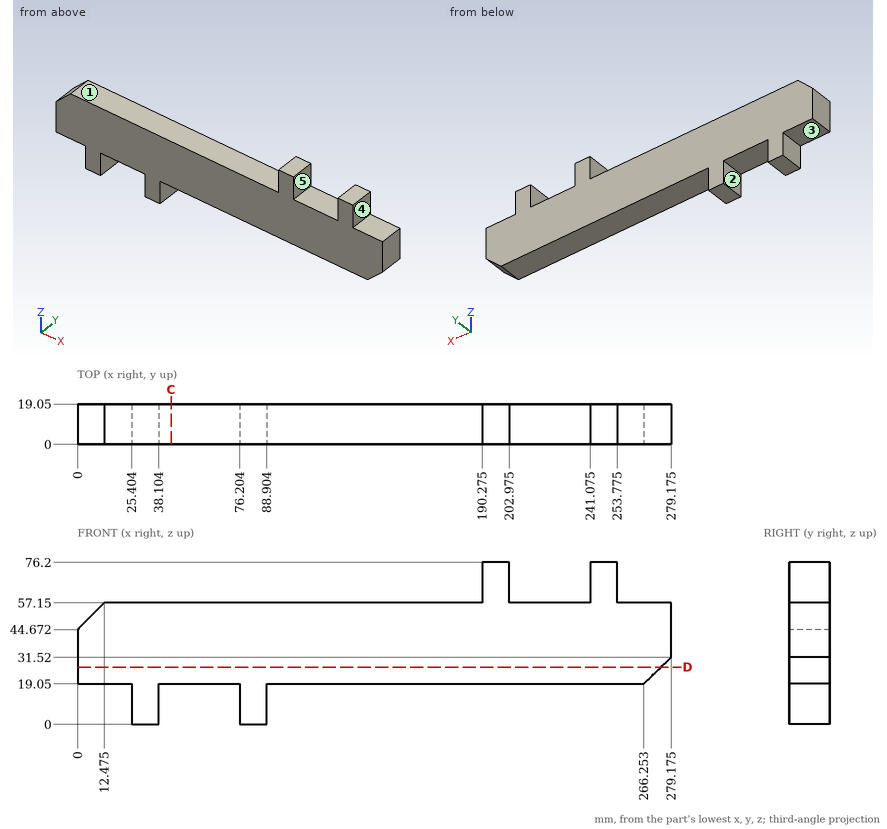
Drawing for the job (mm, zero at the part's lowest x, y, z). A direction names the side the tool comes from. Round coordinates to 2 decimals unless told otherwise and drop trailing zeros. Loops run counter-clockwise (first coordinate to the right, second up) from the corner with the lowest first, then second, coordinate; pieces in that order, holes last.
1. Band-saw the part on D-D, the plane z = 27. List the corners of the cut face in (x, y).
Check values:
outline: (0, 0) - (274.49, 0) - (274.49, 19.05) - (0, 19.05) - close
2. Drop flat-ended pins along their axis: P1, Ø9.5, axis at y = 13.5, z = 65.5, coming from the -X side (1 decimal); P2, Ø5.5, axis at x = 53.5, y = 6.5, coming from the -Z side; P3, Ø9.5, axis at y = 8.5, z = 67, coming from the +X side (1 decimal); P4, Ø5, axis at x = 101, z = 16.5, coming from the +Y side. Give the stop position or say it passes through.
Check values:
P1: stops at x = 190.3
P2: stops at z = 19.05
P3: stops at x = 253.8
P4: passes through
3. Wall check: probe 1 along X at (y, z) = (14.75, 62.5) (1 decimal); probe 2 along X at (y, z) = (17, 13) (1 decimal); probe 3 along Z at (x, y) = (117, 5.25). Give the ranges that are in metal, low to high.
Check values:
probe 1: x = 190.3 to 203, 241.1 to 253.8
probe 2: x = 25.4 to 38.1, 76.2 to 88.9
probe 3: z = 19.05 to 57.15
4. Tool access for the marked faces 1, 2, 3, 4 and 5: list every direction of +Z, -Z, +X, -X, +Y, -Y with a clear straight run to the whole face (end or side of a thin tool).
Check values:
face 1: +Z, -X, +Y, -Y
face 2: -Z, +Y, -Y
face 3: -Z, -X, +Y, -Y
face 4: +Z, +X, +Y, -Y
face 5: +Z, +Y, -Y
5. Band-saw the part on C-C, the plane x = 44. List the corners of the cut face in (y, z).
Check values:
outline: (0, 19.05) - (19.05, 19.05) - (19.05, 57.15) - (0, 57.15) - close
